Here's how the part is built. I have some questions about the finished solid (model axes, mm). A direction names the side the tool comes from. Round coordinates to 2 decimals unless told otherwise and drop trailing zeros. Write each loop counter-clockwise with the first axis right and the second up, starting at its lowest first coordinate (ties: lowest second). Pieces come first, ordered by that corner, then holes. Notation, with made-up numbers: (19.5, 70.5) - (29.5, 70.5) arc R29 ccw to (29.5, 92.5) - close; hole circle Ø7 at (-28, -8.5). An arc over 180 degrees is marked (long way). Return JSON: item names as keys, results as strings. Group by question number.
```python
from build123d import *

# Parameters (mm, degrees)
F0_R      = 9.525
F1_DEPTH  = 12.7
F2_R      = 7.506921
F3_DEPTH  = 25.4
F4_W      = 20.066
F4_H      = 63.5
F5_DEPTH  = 11.684
F5_FACE_R = 7.506921
F6_DEPTH  = 25.4


with BuildPart() as f1:
    # F0 (on Front) → F1 (new body)
    with BuildSketch(Plane.XZ):
        with Locations((-23.762971, 23.442931)):
            Circle(F0_R)
    extrude(amount=F1_DEPTH)

    # F2 (on face) → F3 (cut)
    with BuildSketch(Plane.XZ.offset(12.7)):
        with Locations((-23.762971, 23.442931)):
            Circle(F2_R)
    extrude(amount=-F3_DEPTH, mode=Mode.SUBTRACT)

    # F4 (on Front) → F5 (join)
    with BuildSketch(Plane.XZ):
        with Locations((-23.671666, 23.678257)):
            Rectangle(F4_W, F4_H)
    extrude(amount=-F5_DEPTH)

    # F5_face (on face) → F6 (cut)
    with BuildSketch(Plane(origin=(-23.762971, 0, 23.442931), x_dir=(1, 0, 0), z_dir=(0, -1, 0))):
        Circle(F5_FACE_R)
    extrude(amount=-F6_DEPTH, mode=Mode.SUBTRACT)


solid = f1.part
```
1) If we mould it in two halves opening along Z, with no side actions, what happens to faces 3 (the cylindrical face through (-19.727, -0.679, 29.773)), 4 (the flat face through (-24, 6, -8.072)), 5 (the flat face through (-33.705, 6, 23))? For each: released by +Z, released by -Z, zero draft, split by the parting line, or undercut.
2) Imagine slicing it at A-A (x = -18.25). Please give me the cut outline in (y, z).
3) Will this pin go through, and if not, where does the flat tip stop? pin 1 Ø9 at (x, z) = (-23.76, 23.44) entering from -Y.
4) Imagine slicing it at D-D (z = 42.5). Please give me the cut outline in (x, y), plus the area to 3 significant figures.
5) For faces 1 (the flat face through (-24, 6, 55.428)), 2 (the cylindrical face through (-25.003, -6.261, 32.887)), which set-ups out of +Z, -Z, +X, -X, +Y, -Y let a thin tool reach every point of the face, with its end or its side?
6) Imagine slicing it at C-C (z = 17.5). Please give me the cut outline in (x, y), plus the area to 3 significant figures.
7) I need wall thicknesses on line 1 along Z through (x, y) = (-23.5, -1.25); line 2 along Z through (x, y) = (-23.5, 7.75); line 3 along Y through (x, z) = (-25.5, 13.5). Which ranges of each line are inside material? Lowest first, please.
8) Imagine slicing it at B-B (y = 8). Please give me the cut outline in (x, z).
Results found:
{
 "1": {"face 3": "undercut", "face 4": "released by -Z", "face 5": "zero draft"},
 "2": {"outline": "(-12.7, 15.68) - (0, 15.68) - (0, -8.07) - (11.68, -8.07) - (11.68, 18.35) - (-12.7, 18.35) - close; (-12.7, 28.54) - (11.68, 28.54) - (11.68, 55.43) - (0, 55.43) - (0, 31.21) - (-12.7, 31.21) - close"},
 "3": {"pin 1": "passes through"},
 "4": {"outline": "(-33.7, 0) - (-13.64, 0) - (-13.64, 11.68) - (-33.7, 11.68) - close", "area": "234 mm²"},
 "5": {"face 1": "+Z, +X, -X, +Y, -Y", "face 2": "-Y"},
 "6": {"outline": "(-33.7, 0) - (-31.21, 0) - (-31.21, -12.7) - (-28.35, -12.7) - (-28.35, 11.68) - (-33.7, 11.68) - close; (-19.18, -12.7) - (-16.32, -12.7) - (-16.32, 0) - (-13.64, 0) - (-13.64, 11.68) - (-19.18, 11.68) - close", "area": "200 mm²"},
 "7": {"line 1": "z = 13.92 to 15.94, 30.95 to 32.96", "line 2": "z = -8.07 to 15.94, 30.95 to 55.43", "line 3": "y = 0 to 11.68"},
 "8": {"outline": "(-33.7, -8.07) - (-13.64, -8.07) - (-13.64, 55.43) - (-33.7, 55.43) - close; hole circle Ø15.01 at (-23.76, 23.44)"}
}
